Build history of the part. All positions in model axes, mm. A direction names the side the tool comes from. Give positions to 0.01 mm unless a question says otherwise; leave off trailing zeros. Write each loop counter-clockwise with the first axis right and the second up, starting at its lowest first coordinate (ties: lowest second). Pieces come first, ordered by that corner, then holes. Notation, with made-up numbers: (50.25, 60.25) -> (106.25, 60.25) arc R26 cw to (106.25, 78.25) -> close; hole circle Ø4 at (-32, 82). An arc over 180 degrees is marked (long way). Put each result on its own line as item: value. Start each with the question number.
Item 1: Slice it at B-B, the plane z = -85. List the corners of the cut face in (x, y), plus the area to 3 significant figures.
Item 2: Slice it at A-A, the plane z = 0. List the corners of the cut face in (x, y).
Item 3: Tool access for faces 5 (the flat face through (-54.463, 2.465, 40.105)), 6 (the flat face through (102.1, 2.46, 110.65)): list every direction of +Z, -Z, +X, -X, +Y, -Y with a clear straight run to the whole face (end or side of a thin tool).
Item 4: Two-plate mould, pull along X, no slides. Class faces 1 (the flat face through (2, 5, -28)), 2 (the flat face through (55.13, 2.46, 40.49)), 3 (the flat face through (147.23, 2.46, 32.48)), 4 (the flat face through (82.325, 2.465, 47.409)): pulls with the +X half, pulls with the -X half, needs draft (parallel to the pull), parting line crosses it, or undercut.
Item 5: Slice it at D-D, the plane z = 140. List the corners of the cut face in (x, y).
Item 6: Slice it at C-C, the plane y = 2.1. Give the number of separate pieces and of enclosed holes in the cut face, plus the area to 3 significant figures.
Item 7: Flat gauge pins, fed straight in: pin 1 Ø4.5 at (x, z) = (40, -125) entering from +Y; pin 2 Ø2.5 at (y, z) = (2.5, -109.5) entering from +X; pin 3 Ø3 at (y, z) = (2, -105) entering from +X; pin 4 Ø1.5 at (x, y) = (83.5, 1) entering from +Z. Where does each tip first touch, or does it go through?
Item 8: Drill centre lines: line 1 along Z through (x, y) = (60, 2.95); line 2 along X through (y, z) = (3.7, -71.5); line 3 along X through (y, z) = (2.75, 17.5). Where is each one in solid material? Low to high.
```python
from build123d import *

# Parameters (mm, degrees)
SKETCH1_R           = 2
SKETCH1_R_2         = 4
SKETCH1_R_3         = 7.5
BOSS_EXTRUDE1_DEPTH = 5


with BuildPart() as part:
    # Sketch1 → Boss-Extrude1 (new body)
    with BuildSketch(Plane(origin=(0, 0, 0), x_dir=(1, 0, 0), z_dir=(0, 1, 0))):
        with BuildLine():
            Line((-20, 143.745078664), (-20, 58.745078664))
            ThreePointArc((-20, 58.745078664), (-16.583123952, 47.564738776), (-7.5, 40.204582446))
            Line((-7.5, 40.204582446), (-7.5, 95))
            Line((-7.5, 95), (7.5, 95))
            Line((7.5, 95), (7.5, 40.204582446))
            ThreePointArc((7.5, 40.204582446), (16.583123952, 47.564738776), (20, 58.745078664))
            Line((20, 58.745078664), (20, 143.745078664))
            Line((20, 143.745078664), (70.266296045, 143.745078664))
            ThreePointArc((70.266296045, 143.745078664), (138.564064606, 80), (159.620037815, -11.020141927))
            Line((159.620037815, -11.020141927), (134.486889792, -54.552031256))
            Line((134.486889792, -54.552031256), (60.87473047, -12.052031256))
            ThreePointArc((60.87473047, -12.052031256), (49.483834081, -9.420962772), (38.568189747, -13.607100695))
            Line((38.568189747, -13.607100695), (86.02241336, -41.004809472))
            Line((86.02241336, -41.004809472), (78.52241336, -53.995190528))
            Line((78.52241336, -53.995190528), (31.068189747, -26.597481751))
            ThreePointArc((31.068189747, -26.597481751), (32.900710129, -38.143776005), (40.87473047, -46.693047408))
            Line((40.87473047, -46.693047408), (114.486889792, -89.193047408))
            Line((114.486889792, -89.193047408), (89.353741769, -132.724936737))
            ThreePointArc((89.353741769, -132.724936737), (0, -160), (-89.353741769, -132.724936737))
            Line((-89.353741769, -132.724936737), (-114.486889792, -89.193047408))
            Line((-114.486889792, -89.193047408), (-40.87473047, -46.693047408))
            ThreePointArc((-40.87473047, -46.693047408), (-32.900710129, -38.143776005), (-31.068189747, -26.597481751))
            Line((-31.068189747, -26.597481751), (-78.52241336, -53.995190528))
            Line((-78.52241336, -53.995190528), (-86.02241336, -41.004809472))
            Line((-86.02241336, -41.004809472), (-38.568189747, -13.607100695))
            ThreePointArc((-38.568189747, -13.607100695), (-49.483834081, -9.420962772), (-60.87473047, -12.052031256))
            Line((-60.87473047, -12.052031256), (-134.486889792, -54.552031256))
            Line((-134.486889792, -54.552031256), (-159.620037815, -11.020141927))
            ThreePointArc((-159.620037815, -11.020141927), (-138.564064606, 80), (-70.266296045, 143.745078664))
            Line((-70.266296045, 143.745078664), (-20, 143.745078664))
        make_face()
        with Locations(Location((40, 125, 0), (0, 0, 270))):
            Circle(SKETCH1_R, mode=Mode.SUBTRACT)
        with Locations(Location((40, 95, 0), (0, 0, 270))):
            Circle(SKETCH1_R, mode=Mode.SUBTRACT)
        with Locations(Location((-40, 95, 0), (0, 0, 90))):
            Circle(SKETCH1_R, mode=Mode.SUBTRACT)
        with Locations(Location((-40, 125, 0), (0, 0, 90))):
            Circle(SKETCH1_R, mode=Mode.SUBTRACT)
        with Locations(Location((102.27241336, -12.858983849, 0), (0, 0, 90))):
            Circle(SKETCH1_R, mode=Mode.SUBTRACT)
        with Locations(Location((128.253175473, -27.858983849, 0), (0, 0, 90))):
            Circle(SKETCH1_R, mode=Mode.SUBTRACT)
        with Locations(Location((88.253175473, -97.141016151, 0), (0, 0, 270))):
            Circle(SKETCH1_R, mode=Mode.SUBTRACT)
        with Locations(Location((62.27241336, -82.141016151, 0), (0, 0, 270))):
            Circle(SKETCH1_R, mode=Mode.SUBTRACT)
        with Locations(Location((-62.272413359, -82.141016151, 0), (0, 0, 90))):
            Circle(SKETCH1_R, mode=Mode.SUBTRACT)
        with Locations(Location((-88.253175473, -97.141016151, 0), (0, 0, 90))):
            Circle(SKETCH1_R, mode=Mode.SUBTRACT)
        with Locations(Location((-128.253175473, -27.858983849, 0), (0, 0, 270))):
            Circle(SKETCH1_R, mode=Mode.SUBTRACT)
        with Locations(Location((-102.272413359, -12.858983849, 0), (0, 0, 270))):
            Circle(SKETCH1_R, mode=Mode.SUBTRACT)
        with Locations(Location((0, -140, 0), (0, 0, 270))):
            Circle(SKETCH1_R_2, mode=Mode.SUBTRACT)
        with Locations(Location((-121.24355653, 70, 0), (0, 0, 270))):
            Circle(SKETCH1_R_2, mode=Mode.SUBTRACT)
        with Locations(Location((121.24355653, 70, 0), (0, 0, 270))):
            Circle(SKETCH1_R_2, mode=Mode.SUBTRACT)
        with Locations(Location((0, 0, 0), (0, 0, 270))):
            Circle(SKETCH1_R_3, mode=Mode.SUBTRACT)
    extrude(amount=BOSS_EXTRUDE1_DEPTH)


solid = part.part
```
Values follow:
1. outline: (-135.55, 0) -> (-20, 0) -> (-20, 5) -> (-135.55, 5) -> close; (-7.5, 0) -> (7.5, 0) -> (7.5, 5) -> (-7.5, 5) -> close; (20, 0) -> (135.55, 0) -> (135.55, 5) -> (20, 5) -> close
1. area: 1,230 mm2
2. outline: (-160, 0) -> (-7.5, 0) -> (-7.5, 5) -> (-160, 5) -> close; (7.5, 0) -> (160, 0) -> (160, 5) -> (7.5, 5) -> close
3. face 5: +Y, -Y
3. face 6: +Z, +X, +Y, -Y
4. face 1: needs draft
4. face 2: undercut
4. face 3: pulls with the +X half
4. face 4: undercut
5. outline: (-77.46, 0) -> (-4, 0) -> (-4, 5) -> (-77.46, 5) -> close; (4, 0) -> (77.46, 0) -> (77.46, 5) -> (4, 5) -> close
6. separate pieces: 1
6. enclosed holes: 16
6. area: 65,800 mm2
7. pin 1: y = 5
7. pin 2: x = 117.82
7. pin 3: x = 122.02
7. pin 4: z = 136.94
8. line 1: -143.75 to 11.58, 25.98 to 43.3, 57.74 to 148.32
8. line 2: -143.14 to -124.95, -117.54 to -20, -7.5 to 7.5, 20 to 117.54, 124.95 to 143.14
8. line 3: -155.88 to -70.31, -45.31 to 45.31, 70.31 to 155.88
